For this review, take the finished solid that the model builds, in its own axes (mm). Face numbers are marked on the shaded views. A direction names the side the tool comes from. Round coordinates to 2 decimals unless told otherwise and drop trailing zeros. Write each loop counter-clockwise with the first axis right and the second up, starting at its lowest first coordinate (ties: lowest second). Pieces come first, ordered by that corner, then holes.
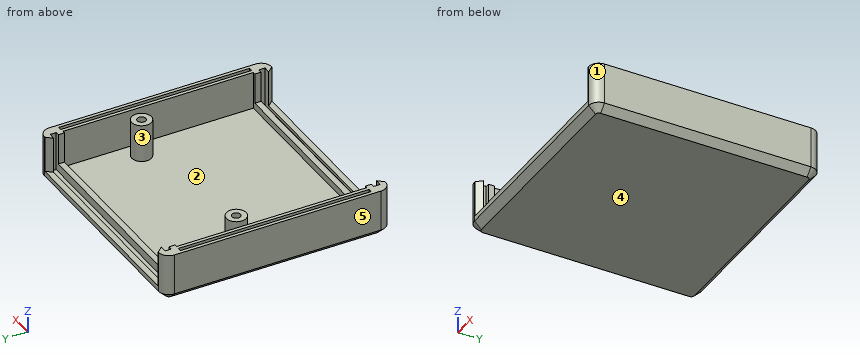
from build123d import *

# Parameters (mm, degrees)
PAD_DEPTH             = 14
SKETCH001_W           = 60
SKETCH001_H           = 55.5
POCKET_DEPTH          = 11
SKETCH002_W           = 60.7
SKETCH002_H           = 1.8
POCKET001_DEPTH       = 11.4
POLARPATTERN_COUNT    = 2
SKETCH003_W           = 58.4
SKETCH003_H           = 2
POCKET002_DEPTH       = 9
POLARPATTERN001_COUNT = 2
POCKET003_DEPTH       = 10.5
POLARPATTERN002_COUNT = 2
SKETCH005_W           = 1.1
SKETCH005_H           = 55.6
POCKET004_DEPTH       = 1.5
POLARPATTERN003_COUNT = 2
SKETCH006_R           = 2.86
SKETCH006_R_2         = 1.25
PAD001_DEPTH          = 11
CHAMFER_SIZE          = 2


with BuildPart() as part:
    # Sketch → Pad (new body)
    with BuildSketch(Plane.XY):
        with BuildLine():
            Line((-33.1, 30.1), (-33.1, -30.1))
            ThreePointArc((-33.1, -30.1), (-32.22132, -32.22132), (-30.1, -33.1))
            Line((-30.1, -33.1), (30.1, -33.1))
            ThreePointArc((30.1, -33.1), (32.22132, -32.22132), (33.1, -30.1))
            Line((33.1, -30.1), (33.1, 30.1))
            ThreePointArc((33.1, 30.1), (32.22132, 32.22132), (30.1, 33.1))
            Line((30.1, 33.1), (-30.1, 33.1))
            ThreePointArc((-30.1, 33.1), (-32.22132, 32.22132), (-33.1, 30.1))
        make_face()
    extrude(amount=PAD_DEPTH)

    # Sketch001 (on DatumPlane) → Pocket (cut)
    with BuildSketch(Plane.XY.offset(14)):
        Rectangle(SKETCH001_W, SKETCH001_H)
    extrude(amount=-POCKET_DEPTH, mode=Mode.SUBTRACT)

    # Sketch002 (on DatumPlane) → Pocket001 (cut)
    with BuildSketch(Plane.XY.offset(14)):
        with Locations((0, 30.45)):
            Rectangle(SKETCH002_W, SKETCH002_H)
    pocket001 = extrude(amount=-POCKET001_DEPTH, mode=Mode.SUBTRACT)

    # PolarPattern: Pocket001 ×2 about axis
    polarpattern_axis = Axis((0, 0, 14), (0, 0, 1))
    for i in range(1, POLARPATTERN_COUNT):
        add(pocket001.rotate(polarpattern_axis, i * 360 / POLARPATTERN_COUNT), mode=Mode.SUBTRACT)

    # Sketch003 (on DatumPlane) → Pocket002 (cut)
    with BuildSketch(Plane.XY.offset(14)):
        with Locations((0, 28.7)):
            Rectangle(SKETCH003_W, SKETCH003_H)
    pocket002 = extrude(amount=-POCKET002_DEPTH, mode=Mode.SUBTRACT)

    # PolarPattern001: Pocket002 ×2 about axis
    polarpattern001_axis = Axis((0, 0, 14), (0, 0, 1))
    for i in range(1, POLARPATTERN001_COUNT):
        add(pocket002.rotate(polarpattern001_axis, i * 360 / POLARPATTERN001_COUNT), mode=Mode.SUBTRACT)

    # Sketch004 (on DatumPlane) → Pocket003 (cut)
    with BuildSketch(Plane.XY.offset(14)):
        Polygon((-28.25, 31.2), (28.25, 31.2), (30, 33.2), (-30, 33.2), align=None)
    pocket003 = extrude(amount=-POCKET003_DEPTH, mode=Mode.SUBTRACT)

    # PolarPattern002: Pocket003 ×2 about axis
    polarpattern002_axis = Axis((0, 0, 14), (0, 0, 1))
    for i in range(1, POLARPATTERN002_COUNT):
        add(pocket003.rotate(polarpattern002_axis, i * 360 / POLARPATTERN002_COUNT), mode=Mode.SUBTRACT)

    # Sketch005 (on DatumPlane) → Pocket004 (cut)
    with BuildSketch(Plane.XY.offset(14)):
        with Locations((-31.55, 0)):
            Rectangle(SKETCH005_W, SKETCH005_H)
    pocket004 = extrude(amount=-POCKET004_DEPTH, mode=Mode.SUBTRACT)

    # PolarPattern003: Pocket004 ×2 about axis
    polarpattern003_axis = Axis((0, 0, 14), (0, 0, 1))
    for i in range(1, POLARPATTERN003_COUNT):
        add(pocket004.rotate(polarpattern003_axis, i * 360 / POLARPATTERN003_COUNT), mode=Mode.SUBTRACT)

    # Sketch006 (on DatumPlane) → Pad001 (join)
    with BuildSketch(Plane.XY.offset(14)):
        with Locations((-25, 7.6)):
            Circle(SKETCH006_R)
        with Locations((-25, 7.6)):
            Circle(SKETCH006_R_2, mode=Mode.SUBTRACT)
        with Locations((25, 7.6)):
            Circle(SKETCH006_R)
        with Locations((25, 7.6)):
            Circle(SKETCH006_R_2, mode=Mode.SUBTRACT)
    extrude(amount=-PAD001_DEPTH)

    # Chamfer
    chamfer_edges = [part.edges().sort_by_distance(p)[0] for p in [
        (0, -33.1, 0),
    ]]
    chamfer(chamfer_edges, length=CHAMFER_SIZE)


solid = part.part
(1) Mouldability with a two-part tool opening along X and no side actions: class the marked faces 3, 4 and 5 as pulls with the +X half, pulls with the -X half, needs draft (parallel to the pull), parting line crosses it, or undercut.
Geometry check:
face 3: undercut
face 4: needs draft
face 5: pulls with the -X half
(2) We need section A-A, the plane x = -5. Give the boundary of the cut face in (y, z), and give its area (3 significant figures).
Geometry check:
outline: (-33.1, 2) - (-31.1, 0) - (31.1, 0) - (33.1, 2) - (33.1, 3.5) - (31.35, 3.5) - (31.35, 2.6) - (29.55, 2.6) - (29.55, 5) - (27.75, 5) - (27.75, 3) - (-27.75, 3) - (-27.75, 5) - (-29.55, 5) - (-29.55, 2.6) - (-31.35, 2.6) - (-31.35, 3.5) - (-33.1, 3.5) - close
area: 202 mm2
(3) For pin 1 Ø1.4 at (x, y) = (12, -28.5) entering from +Z; pin 2 Ø1.2 at (x, z) = (-32, 13.5) entering from -Y; pin 3 Ø5.5 at (x, z) = (8, 7) entering from -Y, all flat-tipped, find the tip position at first contact; note any pin that passes through.
Geometry check:
pin 1: stops at z = 5
pin 2: stops at y = -32.8
pin 3: stops at y = -29.55
(4) We need section C-C, the plane z = 7.75. State how many separate pieces and enclosed holes the cut face has, and give its area (3 significant figures).
Geometry check:
separate pieces: 4
enclosed holes: 2
area: 454 mm2
(5) For the marked faces 1 and 2, list the 3-axis set-ups (+Z, -Z, +X, -X, +Y, -Y) from which the entire face can be reached by the end or side of a thin tool; tool diameter is ignored.
Geometry check:
face 1: +Z, -Z, +X, -Y
face 2: +Z
(6) For line 1 along Y through (x, z) = (25, 6); line 2 along X through (y, z) = (-24, 3.5); line 3 along Y through (x, z) = (6, 4.25), list the stretches that pass through material, from the lowest coordinate up.
Geometry check:
line 1: y = 4.74 to 6.35, 8.85 to 10.46
line 2: x = -33.1 to -30, 30 to 33.1
line 3: y = -29.55 to -27.75, 27.75 to 29.55
(7) We need section D-D, the plane y = -23.5. Give the boundary of the cut face in (x, z), and give its area (4 significant figures).
Geometry check:
outline: (-33.1, 2) - (-31.1, 0) - (31.1, 0) - (33.1, 2) - (33.1, 14) - (32.1, 14) - (32.1, 12.5) - (31, 12.5) - (31, 14) - (30, 14) - (30, 3) - (-30, 3) - (-30, 14) - (-31, 14) - (-31, 12.5) - (-32.1, 12.5) - (-32.1, 14) - (-33.1, 14) - close
area: 259.5 mm2
